Check sheet for the modelled part. Datum: model origin and axes. Units: mm. A direction names the side the tool comes from. Coordinates: 2 decimals unless noted, no trailing zeros. Write each loop counter-clockwise with the first axis right and the second up, starting at its lowest first coordinate (ties: lowest second). Pieces come first, ordered by that corner, then holes. Notation, with made-up numbers: (46, -33) -> (65, -33) arc R30 cw to (65, 6) -> close; hole circle Ø4 at (40.25, 14). An arc over 180 degrees is marked (long way). One line per item, written item: value. Start each with the question number.
1) Sectioned sample at D-D on x = 18. Enter the section's corners in (y, z), plus the area to 3 significant figures.
2) Scan lines: line 1 along Y through (x, z) = (24.25, 1.95); line 2 along X through (y, z) = (2.25, 3.65); line 3 along Z through (x, y) = (-0.85, 11). Record each from-to range of solid material in increasing order. Write a range as [from, to].
3) Sectioned sample at A-A on z = 2.1. Give the number of separate pieces and of enclosed holes in the cut face, plus the area to 3 significant figures.
4) Set-up check for faces 1 (the flat face through (4.25, 0.5, 3)), 2 (the flat face through (24, 23, 1)), 3 (the cylindrical face through (-1.479, 9.235, 3.056)): record each of +Z, -Z, +X, -X, +Y, -Y from which the full face is reachable in a straight line by a thin tool's end or side.
5) Draft check along Y on faces 4 (the flat face through (23.25, 0.5, 3)), 5 (the flat face through (13.6, 0, 0.8)), 6 (the flat face through (25, 12, 4)). Enter one of: +Y half, -Y half, draft (parallel to the pull), parting line (faces both ways), or undercut.
6) Sectioned sample at C-C on x = 3.25. Enter the section's corners in (y, z), plus the area to 3 significant figures.
7) Gauge pin test, flat ends, axial feed: P1, Ø3, axis at x = 24.25, y = 10.75, coming from the +Z side; P2, Ø1, axis at y = 6, z = 4, coming from the -X side; P3, Ø7.5, axis at x = 8.5, y = 7, coming from the +Z side. Record the tip position at first contact, or that the pin passes through.
8) Sectioned sample at B-B on y = 19.25. Enter the section's corners in (x, z), plus the area to 3 significant figures.
```python
from build123d import *

# Parameters (mm, degrees)
SKETCH_W        = 27.5
SKETCH_H        = 26.5
PAD_DEPTH       = 5
SKETCH001_W     = 25.5
SKETCH001_H     = 24.5
POCKET_DEPTH    = 4
SKETCH002_W     = 19
SKETCH002_H     = 4
POCKET001_DEPTH = 1
SKETCH003_R     = 2
SKETCH003_R_2   = 1
PAD001_DEPTH    = 3
SKETCH004_R     = 2.5
SKETCH004_R_2   = 1.85
PAD002_DEPTH    = 3


with BuildPart() as part:
    # Sketch → Pad (new body)
    with BuildSketch(Plane.XY):
        with Locations((13.75, 13.25)):
            Rectangle(SKETCH_W, SKETCH_H)
    extrude(amount=PAD_DEPTH)

    # Sketch001 → Pocket (cut)
    with BuildSketch(Plane.XY.offset(5)):
        with Locations((13.75, 13.25)):
            Rectangle(SKETCH001_W, SKETCH001_H)
    extrude(amount=-POCKET_DEPTH, mode=Mode.SUBTRACT)

    # Sketch002 → Pocket001 (cut)
    with BuildSketch(Plane.XZ):
        with Locations((13.75, 3)):
            Rectangle(SKETCH002_W, SKETCH002_H)
    extrude(amount=-POCKET001_DEPTH, mode=Mode.SUBTRACT)

    # Sketch003 → Pad001 (new body)
    with BuildSketch(Plane.XY.offset(1)):
        with Locations((24.25, 10.75)):
            Circle(SKETCH003_R)
        with Locations((24.25, 10.75)):
            Circle(SKETCH003_R_2, mode=Mode.SUBTRACT)
        with Locations((3.25, 10.75)):
            Circle(SKETCH003_R)
        with Locations((3.25, 10.75)):
            Circle(SKETCH003_R_2, mode=Mode.SUBTRACT)
        with Locations((3.25, 23.25)):
            Circle(SKETCH003_R)
        with Locations((3.25, 23.25)):
            Circle(SKETCH003_R_2, mode=Mode.SUBTRACT)
        with Locations((24.25, 23.25)):
            Circle(SKETCH003_R)
        with Locations((24.25, 23.25)):
            Circle(SKETCH003_R_2, mode=Mode.SUBTRACT)
    extrude(amount=PAD001_DEPTH)

    # Sketch004 → Pad002 (new body)
    with BuildSketch(Plane(origin=(0, 0, 0), x_dir=(0, -1, 0), z_dir=(-1, 0, 0))):
        with Locations((-11, 2.5)):
            Circle(SKETCH004_R)
        with Locations((-11, 2.5)):
            Circle(SKETCH004_R_2, mode=Mode.SUBTRACT)
    extrude(amount=PAD002_DEPTH)


solid = part.part
```
Answers:
1. outline: (0, 0) -> (26.5, 0) -> (26.5, 5) -> (25.5, 5) -> (25.5, 1) -> (0, 1) -> close
1. area: 30.5 mm2
2. line 1: y = [0, 1], [8.75, 9.75], [11.75, 12.75], [21.25, 22.25], [24.25, 25.25], [25.5, 26.5]
2. line 2: x = [0, 1], [26.5, 27.5]
2. line 3: z = [0, 0.65], [4.35, 5]
3. separate pieces: 5
3. enclosed holes: 4
3. area: 127 mm2
4. face 1: +Z, -Y
4. face 2: +Z
4. face 3: -X
5. face 4: draft
5. face 5: -Y half
5. face 6: undercut
6. outline: (0, 0) -> (26.5, 0) -> (26.5, 5) -> (25.5, 5) -> (25.5, 1) -> (25.25, 1) -> (25.25, 4) -> (24.25, 4) -> (24.25, 1) -> (22.25, 1) -> (22.25, 4) -> (21.25, 4) -> (21.25, 1) -> (12.75, 1) -> (12.75, 4) -> (11.75, 4) -> (11.75, 1) -> (9.75, 1) -> (9.75, 4) -> (8.75, 4) -> (8.75, 1) -> (1, 1) -> (1, 5) -> (0, 5) -> close
6. area: 46.5 mm2
7. P1: stops at z = 4
7. P2: stops at x = 0
7. P3: stops at z = 1
8. outline: (0, 0) -> (27.5, 0) -> (27.5, 5) -> (26.5, 5) -> (26.5, 1) -> (1, 1) -> (1, 5) -> (0, 5) -> close
8. area: 35.5 mm2
